Build history of the part. All positions in model axes, mm. A direction names the side the tool comes from. Coordinates: 2 decimals unless noted, no trailing zeros. Loops run counter-clockwise (first coordinate to the right, second up) from the corner with the lowest first, then second, coordinate; pieces in that order, holes last.
(1) Flat gauge pins, fed straight in: P1, Ø4, axis at y = -4, z = 4, coming from the -X side; P2, Ø1.9, axis at y = 10.5, z = 16, coming from the -X side; P3, Ø1.1, axis at y = -4, z = -20, coming from the +X side. Where does each tip first touch, or does it go through?
(2) Slice it at B-B (z = 3.5). Give the cut face in (x, y), and give its area (3 significant figures).
(3) Wall check: L1, parallel to Y at x = -1.75, z = -8; L2, parallel to Z at x = -3.75, y = -3.25; L3, parallel to X at y = 6.75, z = 1. Give the ranges that are in metal, low to high.
(4) Two-plate mould, pull along Z, no slides. Class faces 1 (the face through (-5.15, -5, 9)), 2 (the face through (-2.126, -10.757, -8.92)), 3 (the face through (-0.16, 3.97, -23.5)): pulls with the +Z half, pulls with the -Z half, needs draft (parallel to the pull), parting line crosses it, or undercut.
(5) Slice it at C-C (x = 11). Give the cut face in (y, z), and give its area (3 significant figures).
(6) Tool access for faces 4 (the face through (3.15, -4, -16)), 5 (the face through (0, 4.475, -18)), 6 (the face through (2.65, -11, -6)): list every direction of +Z, -Z, +X, -X, +Y, -Y with a clear straight run to the whole face (end or side of a thin tool).
(7) Slice it at A-A (z = 12). Give the cut face in (x, y) (3 decimals).
from build123d import *

# Parameters (mm, degrees)
BLOCOBASE_DEPTH           = 5
SKFIXACAO_R               = 1.7
SKFIXACAO_R_2             = 1.55
FIXACAO_DEPTH             = 5.15
RESSALTOFIXACAO_DEPTH     = 0.15
BOTAO_DEPTH               = 2.15
SKETCH5_W                 = 6.3
SKETCH5_H                 = 1
BASECONECTORNONC_DEPTH    = 10.5
SKDESENHOCONECTORNONC_R   = 0.75
DESENHOCONECTORNONC_DEPTH = 20.5
BASECONECTORCOM_DEPTH     = 3.15
SKDESENHOCONECTORCOM_R    = 0.75
DESENHOCONECTORCOM_DEPTH  = 1
BASECONTATO_DEPTH         = 3.15
SKAPOIOROLO_R             = 0.7
APOIOROLO_DEPTH           = 1
SKROLO_R                  = 2.5
ROLO_DEPTH                = 4.3
SKETCH6_W                 = 15.037683952
SKETCH6_H                 = 10.848275608
CUT_EXTRUDE1_DEPTH        = 10
SKETCH7_W                 = 16.137668404
SKETCH7_H                 = 7.258990492
BOSS_EXTRUDE1_DEPTH       = 1


with BuildPart() as part:
    # skBlocoBase → BlocoBase (new body, symmetric)
    with BuildSketch(Plane(origin=(0, 0, 0), x_dir=(0, 0, -1), z_dir=(1, 0, 0))):
        with BuildLine():
            Line((-10.7, 7.95), (10.7, 7.95))
            ThreePointArc((10.7, 7.95), (12.9627417, 7.0127417), (13.9, 4.75))
            Line((13.9, 4.75), (13.9, -4.75))
            ThreePointArc((13.9, -4.75), (12.9627417, -7.0127417), (10.7, -7.95))
            Line((10.7, -7.95), (-10.7, -7.95))
            ThreePointArc((-10.7, -7.95), (-12.9627417, -7.0127417), (-13.9, -4.75))
            Line((-13.9, -4.75), (-13.9, 4.75))
            ThreePointArc((-13.9, 4.75), (-12.9627417, 7.0127417), (-10.7, 7.95))
        make_face()
    extrude(amount=BLOCOBASE_DEPTH, both=True)

    # skFixacao → Fixacao (cut, symmetric)
    with BuildSketch(Plane(origin=(0, 0, 0), x_dir=(0, 0, -1), z_dir=(1, 0, 0))):
        with Locations((-11.125, -5.1)):
            Circle(SKFIXACAO_R)
        with Locations((11.125, 5.1)):
            Circle(SKFIXACAO_R_2)
    extrude(amount=FIXACAO_DEPTH, both=True, mode=Mode.SUBTRACT)

    # skRessaltoFixacao → RessaltoFixacao (add)
    with BuildSketch(Plane(origin=(5, 0, 0), x_dir=(0, 0, -1), z_dir=(1, 0, 0))):
        with BuildLine():
            ThreePointArc((-8.475, -5.525), (-9.353679656, -3.403679656), (-11.475, -2.525))
            Line((-11.475, -2.525), (-13.7, -2.525))
            Line((-13.7, -2.525), (-13.7, -4.75))
            ThreePointArc((-13.7, -4.75), (-12.821320344, -6.871320344), (-10.7, -7.75))
            Line((-10.7, -7.75), (-8.475, -7.75))
            Line((-8.475, -7.75), (-8.475, -5.525))
        make_face()
        with BuildLine():
            ThreePointArc((-9.789845005, -6.152312282), (-10.474438165, -6.670595205), (-11.325, -6.788194302))
            ThreePointArc((-11.325, -6.788194302), (-11.775561835, -3.529404795), (-9.789845005, -6.152312282))
        make_face(mode=Mode.SUBTRACT)
        with BuildLine():
            ThreePointArc((13.775, 4.675), (12.896320344, 6.796320344), (10.775, 7.675))
            Line((10.775, 7.675), (8.55, 7.675))
            Line((8.55, 7.675), (8.55, 5.45))
            ThreePointArc((8.55, 5.45), (9.428679656, 3.328679656), (11.55, 2.45))
            Line((11.55, 2.45), (13.775, 2.45))
            Line((13.775, 2.45), (13.775, 4.675))
        make_face()
        with BuildLine():
            ThreePointArc((12.353274612, 4.1545681), (11.71815932, 3.667986725), (10.925, 3.562957385))
            ThreePointArc((10.925, 3.562957385), (10.53184068, 6.532013275), (12.353274612, 4.1545681))
        make_face(mode=Mode.SUBTRACT)
    ressaltofixacao = extrude(amount=RESSALTOFIXACAO_DEPTH)

    # MirrorRessaltoFixacao: RessaltoFixacao across plane
    add(ressaltofixacao.mirror(Plane(origin=(0, 0, 0), x_dir=(0, 0, 1), z_dir=(1, 0, 0))))

    # skBotao → Botao (add, symmetric)
    with BuildSketch(Plane(origin=(0, 0, 0), x_dir=(0, 0, -1), z_dir=(1, 0, 0))):
        with BuildLine():
            Line((-10.475, 7.95), (-10.475, 8.6))
            ThreePointArc((-10.475, 8.6), (-9.075, 9.6), (-7.675, 8.6))
            Line((-7.675, 8.6), (-7.675, 7.95))
            Line((-7.675, 7.95), (-10.475, 7.95))
        make_face()
    extrude(amount=BOTAO_DEPTH, both=True)

    # Sketch5 → BaseConectorNONC (add)
    with BuildSketch(Plane(origin=(0, 0, -13.9), x_dir=(-1, 0, 0), z_dir=(0, 0, -1))):
        with Locations((0, -3.975)):
            Rectangle(SKETCH5_W, SKETCH5_H)
        with Locations((0, 3.975)):
            Rectangle(SKETCH5_W, SKETCH5_H)
    extrude(amount=BASECONECTORNONC_DEPTH)

    # skDesenhoConectorNONC → DesenhoConectorNONC (cut)
    with BuildSketch(Plane.XZ.offset(4.475)):
        Polygon((2.65, -22.767142952), (1.616967042, -24.4), (3.15, -24.4), (3.15, -18.161236833), (2.65, -18.161236833), align=None)
        Polygon((-3.15, -24.4), (-1.616967042, -24.4), (-2.65, -22.767142952), (-2.65, -18.161236833), (-3.15, -18.161236833), align=None)
        with Locations((0, -22.767142952)):
            Circle(SKDESENHOCONECTORNONC_R)
    extrude(amount=-DESENHOCONECTORNONC_DEPTH, mode=Mode.SUBTRACT)

    # skBaseConectorCOM → BaseConectorCOM (add, symmetric)
    with BuildSketch(Plane(origin=(0, 0, 0), x_dir=(0, 0, -1), z_dir=(1, 0, 0))):
        with BuildLine():
            Line((9.725, -11.25), (0.225, -11.25))
            ThreePointArc((0.225, -11.25), (-0.482106781, -10.957106781), (-0.775, -10.25))
            Line((-0.775, -10.25), (-0.775, -7.95))
            Line((-0.775, -7.95), (0.225, -7.95))
            Line((0.225, -7.95), (0.225, -9.25))
            ThreePointArc((0.225, -9.25), (0.517893219, -9.957106781), (1.225, -10.25))
            Line((1.225, -10.25), (9.725, -10.25))
            Line((9.725, -10.25), (9.725, -11.25))
        make_face()
    extrude(amount=BASECONECTORCOM_DEPTH, both=True)

    # skDesenhoConectorCOM → DesenhoConectorCOM (cut)
    with BuildSketch(Plane.XZ.offset(11.25)):
        Polygon((2.65, -8.092142952), (1.616967042, -9.725), (3.15, -9.725), (3.15, -3.486236833), (2.65, -3.486236833), align=None)
        Polygon((-3.15, -9.725), (-1.616967042, -9.725), (-2.65, -8.092142952), (-2.65, -3.486236833), (-3.15, -3.486236833), align=None)
        with Locations((0, -8.092142952)):
            Circle(SKDESENHOCONECTORCOM_R)
    extrude(amount=-DESENHOCONECTORCOM_DEPTH, mode=Mode.SUBTRACT)

    # skBaseContato → BaseContato (add, symmetric)
    with BuildSketch(Plane(origin=(0, 0, 0), x_dir=(0, 0, -1), z_dir=(1, 0, 0))):
        with BuildLine():
            Line((2.63302332, 7.95), (2.63302332, 8.486635004))
            ThreePointArc((2.63302332, 8.486635004), (2.497665983, 8.828739854), (2.164880406, 8.985619098))
            Line((2.164880406, 8.985619098), (-24.4, 10.681624431))
            Line((-24.4, 10.681624431), (-24.336285828, 11.679592619))
            Line((-24.336285828, 11.679592619), (3.545575005, 9.899506131))
            ThreePointArc((3.545575005, 9.899506131), (3.878360582, 9.742626887), (4.013717919, 9.400522037))
            Line((4.013717919, 9.400522037), (4.013717919, 7.95))
            Line((4.013717919, 7.95), (2.63302332, 7.95))
        make_face()
    extrude(amount=BASECONTATO_DEPTH, both=True)

    # skApoioRolo → ApoioRolo (add)
    with BuildSketch(Plane(origin=(3.15, 0, 0), x_dir=(0, 0, -1), z_dir=(1, 0, 0))):
        with BuildLine():
            ThreePointArc((-21.354211514, 14.486814776), (-22.754211514, 15.886814776), (-24.154211514, 14.486814776))
            Line((-24.154211514, 14.486814776), (-24.336285828, 11.679592619))
            Line((-24.336285828, 11.679592619), (-22.939130364, 11.590392778))
            Line((-22.939130364, 11.590392778), (-21.541974901, 11.501192936))
            Line((-21.541974901, 11.501192936), (-21.365242034, 14.3114187))
            Line((-21.365242034, 14.3114187), (-21.354211514, 14.486814776))
        make_face()
        with Locations((-22.754211514, 14.486814776)):
            Circle(SKAPOIOROLO_R, mode=Mode.SUBTRACT)
    apoiorolo = extrude(amount=-APOIOROLO_DEPTH)

    # MirrorApoioRolo: ApoioRolo across plane
    add(apoiorolo.mirror(Plane(origin=(0, 0, 0), x_dir=(0, 0, 1), z_dir=(1, 0, 0))))

    # skRolo → Rolo (add)
    with BuildSketch(Plane.ZY.offset(-2.15)):
        with Locations((22.754211514, 14.486814776)):
            Circle(SKROLO_R)
    extrude(amount=ROLO_DEPTH)

    # Sketch6 → Cut-Extrude1 (cut)
    with BuildSketch(Plane(origin=(0, 10.084763511, -0.643850544), x_dir=(1, 0, 0), z_dir=(0, 0.997968188, -0.063714172))):
        with Locations((-4.368841976, -23.671158356)):
            Rectangle(SKETCH6_W, SKETCH6_H)
    extrude(amount=CUT_EXTRUDE1_DEPTH, mode=Mode.SUBTRACT)

    # Sketch7 → Boss-Extrude1 (add)
    with BuildSketch(Plane(origin=(0, 9.086795323, -0.580136372), x_dir=(1, 0, 0), z_dir=(0, -0.997968188, 0.063714172))):
        with Locations((4.918834202, 21.401499401)):
            Rectangle(SKETCH7_W, SKETCH7_H)
    extrude(amount=BOSS_EXTRUDE1_DEPTH)


solid = part.part
Response values:
1. P1: stops at x = -5
1. P2: stops at x = -3.15
1. P3: stops at x = 2.65
2. outline: (-5, -7.95) - (5, -7.95) - (5, 7.95) - (-5, 7.95) - close; (-3.15, 9.35) - (3.15, 9.35) - (3.15, 10.35) - (-3.15, 10.35) - close
2. area: 165 mm2
3. L1: y = -11.25 to -10.25, -7.95 to 7.95
3. L2: z = -13.9 to 13.9
3. L3: x = -5 to 5
4. face 1: needs draft
4. face 2: pulls with the -Z half
4. face 3: undercut
5. outline: (9.22, 17.22) - (10.22, 17.16) - (10.68, 24.4) - (9.68, 24.46) - close
5. area: 7.26 mm2
6. face 4: -Z, +X, +Y, -Y
6. face 5: -Z, +X, -X, +Y
6. face 6: -Z, +X, -Y
7. outline: (-5.15, -7.454) - (-5, -7.454) - (-5, -7.674) - (5, -7.674) - (5, -7.454) - (5.15, -7.454) - (5.15, -6.558) - (-5.15, -6.558) - close; (-5.15, -3.642) - (5.15, -3.642) - (5.15, -2.525) - (5, -2.525) - (5, 7.674) - (-5, 7.674) - (-5, -2.525) - (-5.15, -2.525) - close; (-3.15, 9.89) - (3.15, 9.89) - (3.15, 10.892) - (-3.15, 10.892) - close
